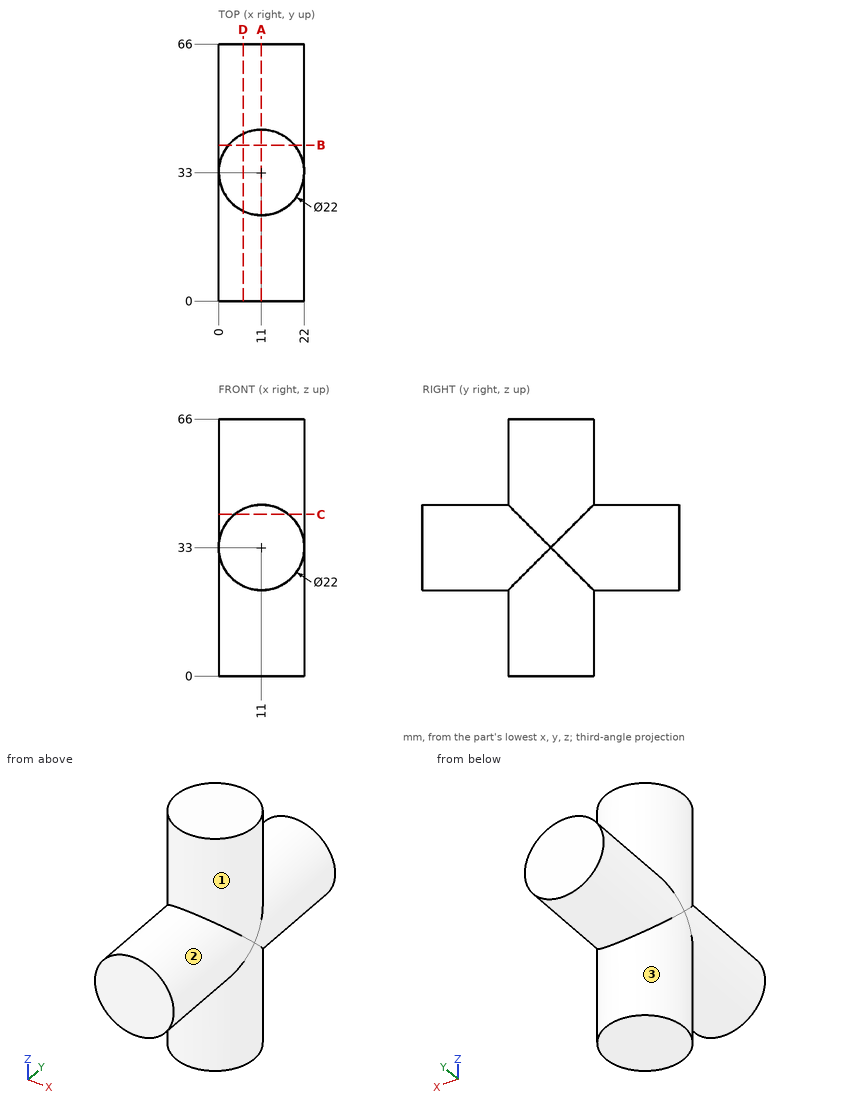
Job drawing, mm, ordinate dimensions from the low corner. One solid piece. A direction names the side the tool comes from. Coordinates: 2 decimals unless noted, no trailing zeros. Write each loop counter-clockwise with the first axis right and the second up, starting at its lowest first coordinate (ties: lowest second). Pieces come first, ordered by that corner, then holes. Notation, with made-up numbers: (34.25, -18) - (68.25, -18) arc R19 ccw to (68.25, 12) - close; hole circle Ø4 at (14, 77). An arc over 180 degrees is marked (long way). Use a Markdown table: item, result. Add a question column.
Item 1: Band-saw the part on A-A, the plane x = 11. Give the cut face in (y, z).
Item 2: Band-saw the part on C-C, the plane z = 41.5. Give the cut face in (x, y), and give its area (3 significant figures).
Item 3: Flat gauge pins, fed straight in: pin 1 (1 mm diameter, centred on x = 7, z = 47, fed in from -Y); pin 2 (5 mm diameter, centred on y = 41.5, z = 39, fed in from +X); pin 3 (1.5 mm diameter, centred on x = 10, z = 20, fed in from -Y). Where does each tip first touch, or does it go through?
Item 4: Band-saw the part on B-B, the plane y = 40. Give the cut face in (x, z), and give its area (3 significant figures).
Item 5: Drill centre lines: L1, parallel to Z at x = 11.25, y = 10; L2, parallel to Y at x = 21, z = 9.5; L3, parallel to X at y = 31, z = 4. Where is each one in solid material? Low to high. Write a range as from..to.
Item 6: Band-saw the part on D-D, the plane x = 6.25. Give the cut face in (y, z).
Item 7: 3-axis set-ups, long thin cutter, end or side, ignore diameter. For the marked faces 1, 2 and 3: which of +Z, -Z, +X, -X, +Y, -Y reach the whole face in a straight line?
Numbers:
| question | item | result |
|---|---|---|
| 1 | outline | (0, 22) - (22, 22) - (22, 0) - (44, 0) - (44, 22) - (66, 22) - (66, 44) - (44, 44) - (44, 66) - (22, 66) - (22, 44) - (0, 44) - close |
| 2 | outline | (4.02, 0) - (17.98, 0) - (17.98, 24.5) arc R11 ccw to (17.98, 41.5) - (17.98, 66) - (4.02, 66) - (4.02, 41.5) arc R11 ccw to (4.02, 24.5) - close |
| 2 | area | 1,020 mm2 |
| 3 | pin 1 | y = 22.57 |
| 3 | pin 2 | x = 21.43 |
| 3 | pin 3 | y = 22 |
| 4 | outline | (2.51, 0) - (19.49, 0) - (19.49, 26) arc R11 ccw to (19.49, 40) - (19.49, 66) - (2.51, 66) - (2.51, 40) arc R11 ccw to (2.51, 26) - close |
| 4 | area | 1,170 mm2 |
| 5 | L1 | 22..44 |
| 5 | L2 | 28.42..37.58 |
| 5 | L3 | 0.18..21.82 |
| 6 | outline | (0, 23.08) - (23.08, 23.08) - (23.08, 0) - (42.92, 0) - (42.92, 23.08) - (66, 23.08) - (66, 42.92) - (42.92, 42.92) - (42.92, 66) - (23.08, 66) - (23.08, 42.92) - (0, 42.92) - close |
| 7 | face 1 | +Z |
| 7 | face 2 | -Y |
| 7 | face 3 | -Z |
